The model under review builds one solid part; all positions refer to its coordinate system, in mm. A direction names the side the tool comes from. Coordinates: 2 decimals unless noted, no trailing zeros. Loops run counter-clockwise (first coordinate to the right, second up) from the corner with the lowest first, then second, coordinate; pieces in that order, holes last. Notation, with made-up numbers: (62.5, 54.5) - (96.5, 54.5) arc R25 ccw to (96.5, 80.5) - close; hole circle Ø9 at (-38, 68). An arc over 180 degrees is marked (long way). Answer in a Markdown table with one row per item. Add a question column.
(1) We need section A-A on x = 21.5. Write out the cut boundary in (y, z), plus the area to 3 significant figures.
(2) Mouldability with a two-part tool opening along Y and no side actions: class faces 3 (the cylindrical face through (6.907, -15.219, 14.79)), 4 (the flat face through (4.8, -1.7, 30)), 5 (the flat face through (19, -25, 15)) as +Y half, -Y half, draft (parallel to the pull), parting line (faces both ways), or undercut.
(3) We need section B-B on z = 26.25. Write out the cut boundary in (x, y), plus the area to 3 significant figures.
(4) We need section C-C on x = 15.5. Write out the cut boundary in (y, z).
(5) For line 1 along X through (y, z) = (-6, 8); line 2 along Y through (x, z) = (32, 3.75); line 3 along Y through (x, z) = (8, 11), list the stretches that pass through material, from the lowest coordinate up.
(6) We need section D-D on y = -4. Write out the cut boundary in (x, z).
(7) For P1, Ø12, axis at y = -14.5, z = 7.5, coming from the +X side; P2, Ø6.5, axis at y = -5, z = 18, coming from the +X side; P3, Ø4, axis at x = 22.5, y = -15, coming from the -Z side, all flat-tipped, find the tip position at first contact; note any pin that passes through.
(8) Machinability: for faces 1 (the flat face through (4.8, -1.7, 0)), 2 (the cylindrical face through (37.096, 20.404, 14.79)), which of the approach directions +Z, -Z, +X, -X, +Y, -Y give a long, thin tool a straight path to every point of the face, cutting with its end or side? Answer none if there is none.
Autodesk Inventor part; units mm, degrees
ref_plane "Начальная плоскость" through (0, 0, 0) normal (0, 0, 1) x (1, 0, 0)
ref_plane "Конечная плоскость" through (0, 0, 30) normal (0, 0, 1) x (1, 0, 0)
ref_plane "YZ Plane" through (0, 0, 0) normal (1, 0, 0) x (0, 1, 0)
ref_plane "Начальная плоскость" through (0, 0, 0) normal (0, 0, 1) x (1, 0, 0)
ref_plane "Конечная плоскость" through (0, 0, 30) normal (0, 0, 1) x (1, 0, 0)
sketch "Эскиз" plane through (0, 0, 0) normal (0, 0, 1) x (1, 0, 0)
  line L0 (0, 0) -> (0, 25)
  line L1 (0, 25) -> (38, 25)
  line L2 (38, 25) -> (38, 22.7512)
  line L3 (34.7791, 19.2623) -> (11.4418, 17.3953)
  line L4 (5, 10.4176) -> (5, 0)
  line L5 (5, 0) -> (0, 0) construction
  line L6 (19, 25) -> (19, 18) construction
  line L7 (38, 19.52) -> (38, 18) construction
  line L8 (38, 18) -> (19, 18) construction
  line L9 (0, 15) -> (0, -27) construction
  line L10 (-5.539, 0) -> (16.0067, 0) construction
  line L11 (0, 0) -> (0, -25)
  line L12 (0, -25) -> (38, -25)
  line L13 (38, -25) -> (38, -22.7512)
  line L14 (34.7791, -19.2623) -> (11.4418, -17.3953)
  line L15 (5, -10.4176) -> (5, 0)
  arc A0 (11.4418, 17.3953) -> (5, 10.4176) centre (12, 10.4176) ccw
  arc A1 (5, -10.4176) -> (11.4418, -17.3953) centre (12, -10.4176) ccw
  arc A2 (34.7791, 19.2623) -> (38, 22.7512) centre (34.5, 22.7512) ccw
  arc A3 (38, -22.7512) -> (34.7791, -19.2623) centre (34.5, -22.7512) ccw
  line L16 (0, 23.4) -> (0, -35.4) construction
  line L17 (-9.8481, 0) -> (20.3158, 0) construction
  point P0 (5, 16.88)
  point P1 (38, -19.52)
  point P2 (5, -16.88)
  point P3 (19, -25)
  point P4 (19, -18)
  dimension "d0" = 5
  dimension "d1" = 25
  dimension "d2" = 38
  dimension "d3" = 7
  dimension "d4" = 19
  dimension "d5" = 1.52
  dimension "d23" = 7
  dimension "d24" = 3.5
  dimension "d25" = 0
extrude "Базовый элемент" add sketch "Эскиз" along normal up to surface (30 mm away) from surface at 0
sketch "Sketch3" plane through (0, 0, 0) normal (0, 0, 1) x (1, 0, 0)
  line L0 (0, 0) -> (10, 0)
ref_plane "Work Plane3" through (0, 0, 0) normal (0, -1, 0) x (1, 0, 0)
sketch "Sketch4" plane through (0, 0, 0) normal (0, -1, 0) x (1, 0, 0)
  line L0 (-2, 0) -> (12, 0)
  line L1 (-2, 30) -> (12, 30)
  dimension "d29" = 30
equation "\"d0\" = G_T"
equation "\"d1\" = 0.5 * G_H"
equation "\"d2\" = G_W"
equation "\"d3\" = G_T1"
equation "\"d4\" = G_C"
equation "\"d23\" = G_IR"
equation "\"d24\" = G_ER"
equation "\"d6\" = G_L"
equation "\"G_W\" = 38"
equation "\"G_T\" = 5"
equation "\"G_T1\" = 7"
equation "\"G_NG\" = 0.08"
equation "\"G_ER\" = 3.5"
equation "\"G_IR\" = 7"
equation "\"G_C\" = 19"
equation "\"G_L\" = d29"
equation "\"ex\" = 0"
equation "\"G_OFFSET_START\" = 0"
equation "\"G_OFFSET_END\" = 0"
properties part number "DIN1026-1 - U 50 - 30" material "Сталь, мягкая"
Outcome:
| question | item | result |
|---|---|---|
| 1 | outline | (-25, 0) - (-18.2, 0) - (-18.2, 30) - (-25, 30) - close; (18.2, 0) - (25, 0) - (25, 30) - (18.2, 30) - close |
| 1 | area | 408 mm² |
| 2 | face 3 | undercut |
| 2 | face 4 | draft |
| 2 | face 5 | -Y half |
| 3 | outline | (0, -25) - (38, -25) - (38, -22.75) arc R3.5 ccw to (34.78, -19.26) - (11.44, -17.4) arc R7 cw to (5, -10.42) - (5, 10.42) arc R7 cw to (11.44, 17.4) - (34.78, 19.26) arc R3.5 ccw to (38, 22.75) - (38, 25) - (0, 25) - close |
| 3 | area | 712 mm² |
| 4 | outline | (-25, 0) - (-17.72, 0) - (-17.72, 30) - (-25, 30) - close; (17.72, 0) - (25, 0) - (25, 30) - (17.72, 30) - close |
| 5 | line 1 | 0 to 5 |
| 5 | line 2 | -25 to -19.04, 19.04 to 25 |
| 5 | line 3 | -25 to -16.16, 16.16 to 25 |
| 6 | outline | (0, 0) - (5, 0) - (5, 30) - (0, 30) - close |
| 7 | P1 | x = 37.18 |
| 7 | P2 | x = 5 |
| 7 | P3 | through |
| 8 | face 1 | -Z, +X, -X, +Y, -Y |
| 8 | face 2 | +Z, -Z, +X |
